Read the model definition and answer for the solid it produces. Units are mm, in the model's axes. Face numbers are marked on the shaded views. A direction names the side the tool comes from. Give positions to 0.01 mm unless a question says otherwise; leave off trailing zeros. Write each loop counter-clockwise with the first axis right and the second up, starting at its lowest first coordinate (ties: lowest second). Pieces come first, ordered by that corner, then holes. Notation, with made-up numbers: (85, -31) -> (131, -31) arc R5 ccw to (131, -22) -> close; hole circle Ø2 at (-27.5, 12.25). An arc over 180 degrees is marked (long way). Answer as CSV lines item,"result". Start each with the question number.
1. Given pin 1 (3 mm diameter, centred on x = 17.5, y = -2, fed in from +Z); pin 2 (1 mm diameter, centred on x = -26, z = -35.5, fed in from -Y); pin 3 (2 mm diameter, centred on y = -30.5, z = -18, fed in from +X); pin 4 (5 mm diameter, centred on x = 1, y = -1, fed in from -Z), each flat-ended and moving along its own axis, determine where each tip first touches the part or whether it passes through.
2. The part is cut by section A-A, the plane z = -35. Determine the outline of the cut face in (x, y).
3. A tool of negligible diameter and unlimited length cuts with its end or side. For the marked faces 1, 2 and 3, from which of +Z, -Z, +X, -X, +Y, -Y can it reach the whole face along a straight path? Write none if from no direction.
4. The part is cut by section B-B, the plane x = 0. Give the number of separate pieces and of enclosed holes in the cut face, and give its area (3 significant figures).
5. For a pull along Y with two mould halves and no side action, classify the marked faces 4, 5 and 6 as pulls with the +Y half, pulls with the -Y half, needs draft (parallel to the pull), parting line crosses it, or undercut.
6. Find the intervals of material crossed by line 1 (Y direction, x = 0, z = -42.05) (3 decimals); line 2 (Y direction, x = 0, z = -45.2); line 3 (X direction, y = 6.5, z = -10), in increasing order.
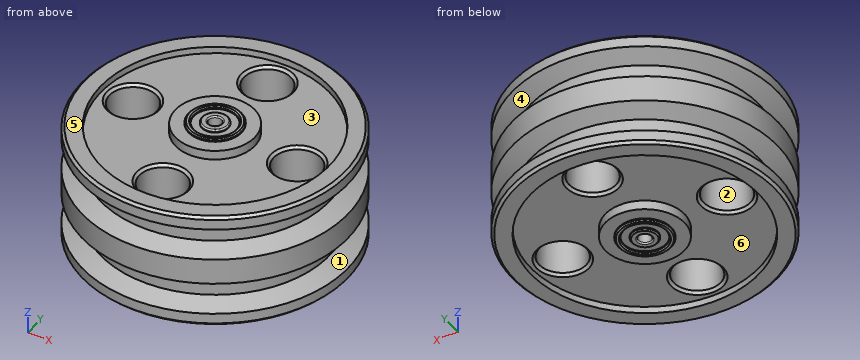
from build123d import *

# Parameters (mm, degrees)
SKETCH2_R            = 50.165
BOSS_EXTRUDE1_DEPTH  = 10
SKETCH4_R            = 43.18
BOSS_EXTRUDE2_DEPTH  = 2
SKETCH5_R            = 50.165
BOSS_EXTRUDE3_DEPTH  = 20
SKETCH7_R            = 43.18
BOSS_EXTRUDE4_DEPTH  = 2
SKETCH8_R            = 50.165
BOSS_EXTRUDE5_DEPTH  = 10
CHAMFER1_SIZE        = 14
CHAMFER1_SIZE_2      = 5.09558328
CHAMFER2_SIZE        = 5.09558328
CHAMFER2_SIZE_2      = 14
CHAMFER4_SIZE        = 14
CHAMFER4_SIZE_2      = 5.09558328
CHAMFER5_SIZE        = 5.09558328
CHAMFER5_SIZE_2      = 14
SKETCH13_R           = 43.18
CUT_EXTRUDE3_DEPTH   = 2.54
SKETCH18_R           = 15
BOSS_EXTRUDE12_DEPTH = 3.5
SKETCH19_R           = 10
BOSS_EXTRUDE13_DEPTH = 1
SKETCH20_R           = 8
SKETCH20_R_2         = 5
CUT_EXTRUDE4_DEPTH   = 1
CUT_EXTRUDE5_START   = -2.54
SKETCH22_R           = 43.18
SKETCH22_R_2         = 15
CUT_EXTRUDE5_DEPTH   = 2.54
SKETCH23_R           = 15
BOSS_EXTRUDE14_DEPTH = 1
BOSS_EXTRUDE15_START = 1
SKETCH24_R           = 10
BOSS_EXTRUDE15_DEPTH = 1
CUT_EXTRUDE6_START   = -1
SKETCH25_R           = 8
SKETCH25_R_2         = 5
CUT_EXTRUDE6_DEPTH   = 1
SKETCH26_R           = 2.5
CUT_EXTRUDE7_DEPTH   = 86.634199068
CHAMFER9_SIZE        = 0.5
FILLET1_R            = 0.5
FILLET2_R            = 0.5
CHAMFER10_SIZE       = 0.5
CHAMFER11_SIZE       = 0.5
FILLET3_R            = 0.5
SKETCH29_R           = 8.89
CUT_EXTRUDE9_DEPTH   = 85.530326215
CHAMFER12_SIZE       = 1
CHAMFER13_SIZE       = 1


with BuildPart() as part:
    # Sketch2 → Boss-Extrude1 (new body)
    with BuildSketch(Plane.XY):
        Circle(SKETCH2_R)
    extrude(amount=-BOSS_EXTRUDE1_DEPTH)

    # Sketch4 → Boss-Extrude2 (add)
    with BuildSketch(Plane(origin=(0, 0, -10), x_dir=(-1, 0, 0), z_dir=(0, 0, -1))):
        with Locations(Location((0, 0, 0), (0, 0, 180))):
            Circle(SKETCH4_R)
    extrude(amount=BOSS_EXTRUDE2_DEPTH)

    # Sketch5 → Boss-Extrude3 (add)
    with BuildSketch(Plane(origin=(0, 0, -12), x_dir=(-1, 0, 0), z_dir=(0, 0, -1))):
        with Locations(Location((0, 0, 0), (0, 0, 180))):
            Circle(SKETCH5_R)
    extrude(amount=BOSS_EXTRUDE3_DEPTH)

    # Sketch7 → Boss-Extrude4 (add)
    with BuildSketch(Plane(origin=(0, 0, -32), x_dir=(-1, 0, 0), z_dir=(0, 0, -1))):
        with Locations(Location((0, 0, 0), (0, 0, 180))):
            Circle(SKETCH7_R)
    extrude(amount=BOSS_EXTRUDE4_DEPTH)

    # Sketch8 → Boss-Extrude5 (add)
    with BuildSketch(Plane(origin=(0, 0, -34), x_dir=(-1, 0, 0), z_dir=(0, 0, -1))):
        with Locations(Location((0, 0, 0), (0, 0, 180))):
            Circle(SKETCH8_R)
    extrude(amount=BOSS_EXTRUDE5_DEPTH)

    # Chamfer1
    # the kernel refuses this chamfer: 14, 5.09558328 mm, written as the material it takes off along each edge
    with BuildSketch(Plane(origin=(0, 0, -10), x_dir=(1, 0, 0), z_dir=(0, -1, 0))) as chamfer1_piece_1_section:
        Polygon((50.165 - CHAMFER1_SIZE, 0), (50.165, CHAMFER1_SIZE_2), (50.165, 0), align=None)
    chamfer1_piece_1 = revolve(axis=Axis((0, 0, -10), (0, 0, 1)), mode=Mode.PRIVATE)
    chamfer1_piece_1 = chamfer1_piece_1 - Plane(origin=(0, 0, -6.275641512), x_dir=(1, 0, 0), z_dir=(0, 0, 1)) * Cylinder(43.18, 201, mode=Mode.PRIVATE)
    add(chamfer1_piece_1, mode=Mode.SUBTRACT)

    # Chamfer2
    # the kernel refuses this chamfer: 14, 5.09558328 mm, written as the material it takes off along each edge
    with BuildSketch(Plane(origin=(0, 0, -12), x_dir=(1, 0, 0), z_dir=(0, 1, 0))) as chamfer2_piece_1_section:
        Polygon((50.165, CHAMFER2_SIZE), (50.165 - CHAMFER2_SIZE_2, 0), (50.165, 0), align=None)
    chamfer2_piece_1 = revolve(axis=Axis((0, 0, -12), (0, 0, -1)), mode=Mode.PRIVATE)
    chamfer2_piece_1 = chamfer2_piece_1 - Plane(origin=(0, 0, -15.724358488), x_dir=(1, 0, 0), z_dir=(0, 0, 1)) * Cylinder(43.18, 201, mode=Mode.PRIVATE)
    add(chamfer2_piece_1, mode=Mode.SUBTRACT)

    # Chamfer4
    # the kernel refuses this chamfer: 14, 5.09558328 mm, written as the material it takes off along each edge
    with BuildSketch(Plane(origin=(0, 0, -32), x_dir=(1, 0, 0), z_dir=(0, 1, 0))) as chamfer4_piece_1_section:
        Polygon((50.165 - CHAMFER4_SIZE, 0), (50.165, -CHAMFER4_SIZE_2), (50.165, 0), align=None)
    chamfer4_piece_1 = revolve(axis=Axis((0, 0, -32), (0, 0, -1)), mode=Mode.PRIVATE)
    chamfer4_piece_1 = chamfer4_piece_1 - Plane(origin=(0, 0, -28.275641512), x_dir=(1, 0, 0), z_dir=(0, 0, 1)) * Cylinder(43.18, 201, mode=Mode.PRIVATE)
    add(chamfer4_piece_1, mode=Mode.SUBTRACT)

    # Chamfer5
    # the kernel refuses this chamfer: 14, 5.09558328 mm, written as the material it takes off along each edge
    with BuildSketch(Plane(origin=(0, 0, -34), x_dir=(1, 0, 0), z_dir=(0, 1, 0))) as chamfer5_piece_1_section:
        Polygon((50.165, CHAMFER5_SIZE), (50.165 - CHAMFER5_SIZE_2, 0), (50.165, 0), align=None)
    chamfer5_piece_1 = revolve(axis=Axis((0, 0, -34), (0, 0, -1)), mode=Mode.PRIVATE)
    chamfer5_piece_1 = chamfer5_piece_1 - Plane(origin=(0, 0, -37.724358488), x_dir=(1, 0, 0), z_dir=(0, 0, 1)) * Cylinder(43.18, 201, mode=Mode.PRIVATE)
    add(chamfer5_piece_1, mode=Mode.SUBTRACT)

    # Sketch13 → Cut-Extrude3 (cut)
    with BuildSketch(Plane.XY):
        Circle(SKETCH13_R)
    extrude(amount=-CUT_EXTRUDE3_DEPTH, mode=Mode.SUBTRACT)

    # Sketch18 → Boss-Extrude12 (add)
    with BuildSketch(Plane.XY.offset(-2.54)):
        Circle(SKETCH18_R)
    extrude(amount=BOSS_EXTRUDE12_DEPTH)

    # Sketch19 → Boss-Extrude13 (add)
    with BuildSketch(Plane.XY.offset(0.96)):
        Circle(SKETCH19_R)
    extrude(amount=BOSS_EXTRUDE13_DEPTH)

    # Sketch20 → Cut-Extrude4 (cut)
    with BuildSketch(Plane.XY.offset(1.96)):
        Circle(SKETCH20_R)
        Circle(SKETCH20_R_2, mode=Mode.SUBTRACT)
    extrude(amount=-CUT_EXTRUDE4_DEPTH, mode=Mode.SUBTRACT)

    # Sketch22 → Cut-Extrude5 (cut)
    with BuildSketch(Plane(origin=(0, 0, -44), x_dir=(-1, 0, 0), z_dir=(0, 0, -1)).offset(CUT_EXTRUDE5_START)):
        with Locations(Location((0, 0, 0), (0, 0, 180))):
            Circle(SKETCH22_R)
        with Locations(Location((0, 0, 0), (0, 0, 180))):
            Circle(SKETCH22_R_2, mode=Mode.SUBTRACT)
    extrude(amount=CUT_EXTRUDE5_DEPTH, mode=Mode.SUBTRACT)

    # Sketch23 → Boss-Extrude14 (add)
    with BuildSketch(Plane(origin=(0, 0, -44), x_dir=(-1, 0, 0), z_dir=(0, 0, -1))):
        with Locations(Location((0, 0, 0), (0, 0, 180))):
            Circle(SKETCH23_R)
    extrude(amount=BOSS_EXTRUDE14_DEPTH)

    # Sketch24 → Boss-Extrude15 (add)
    with BuildSketch(Plane(origin=(0, 0, -45), x_dir=(-1, 0, 0), z_dir=(0, 0, -1)).offset(BOSS_EXTRUDE15_START)):
        with Locations(Location((0, 0, 0), (0, 0, 180))):
            Circle(SKETCH24_R)
    extrude(amount=-BOSS_EXTRUDE15_DEPTH)

    # Sketch25 → Cut-Extrude6 (cut)
    with BuildSketch(Plane(origin=(0, 0, -46), x_dir=(-1, 0, 0), z_dir=(0, 0, -1)).offset(CUT_EXTRUDE6_START)):
        with Locations(Location((0, 0, 0), (0, 0, 180))):
            Circle(SKETCH25_R)
        with Locations(Location((0, 0, 0), (0, 0, 180))):
            Circle(SKETCH25_R_2, mode=Mode.SUBTRACT)
    extrude(amount=CUT_EXTRUDE6_DEPTH, mode=Mode.SUBTRACT)

    # Sketch26 → Cut-Extrude7 (cut, through all)
    with BuildSketch(Plane.XY.offset(1.96)):
        Circle(SKETCH26_R)
    extrude(amount=-CUT_EXTRUDE7_DEPTH, mode=Mode.SUBTRACT)

    # Chamfer9
    chamfer9_edges = [part.edges().sort_by_distance(p)[0] for p in [
        (-10, 0, 1.96),
        (-8, 0, 1.96),
    ]]
    chamfer(chamfer9_edges, length=CHAMFER9_SIZE)

    # Fillet1
    fillet1_edges = [part.edges().sort_by_distance(p)[0] for p in [
        (-5, 0, 1.96),
    ]]
    fillet(fillet1_edges, radius=FILLET1_R)

    # Fillet2
    fillet2_edges = [part.edges().sort_by_distance(p)[0] for p in [
        (-2.5, 0, 1.96),
    ]]
    fillet(fillet2_edges, radius=FILLET2_R)

    # Chamfer10
    chamfer10_edges = [part.edges().sort_by_distance(p)[0] for p in [
        (-10, 0, -46),
        (-8, 0, -46),
    ]]
    chamfer(chamfer10_edges, length=CHAMFER10_SIZE)

    # Chamfer11
    chamfer11_edges = [part.edges().sort_by_distance(p)[0] for p in [
        (-5, 0, -46),
    ]]
    chamfer(chamfer11_edges, length=CHAMFER11_SIZE)

    # Fillet3
    fillet3_edges = [part.edges().sort_by_distance(p)[0] for p in [
        (-2.5, 0, -46),
    ]]
    fillet(fillet3_edges, radius=FILLET3_R)

    # Sketch29 → Cut-Extrude9 (cut, through all)
    with BuildSketch(Plane(origin=(0, 0, -44), x_dir=(-1, 0, 0), z_dir=(0, 0, -1))):
        with Locations((0, 31.75)):
            Circle(SKETCH29_R)
        with Locations((31.75, 0)):
            Circle(SKETCH29_R)
        with Locations((0, -31.75)):
            Circle(SKETCH29_R)
        with Locations((-31.75, 0)):
            Circle(SKETCH29_R)
    extrude(amount=-CUT_EXTRUDE9_DEPTH, mode=Mode.SUBTRACT)

    # Chamfer12
    chamfer12_edges = [part.edges().sort_by_distance(p)[0] for p in [
        (8.89, 31.75, -2.54),
        (8.89, 31.75, -41.46),
        (-22.86, 0, -2.54),
        (-22.86, 0, -41.46),
        (8.89, -31.75, -2.54),
        (8.89, -31.75, -41.46),
        (40.64, 0, -2.54),
        (40.64, 0, -41.46),
    ]]
    chamfer(chamfer12_edges, length=CHAMFER12_SIZE)

    # Chamfer13
    chamfer13_edges = [part.edges().sort_by_distance(p)[0] for p in [
        (-50.165, 0, 0),
        (-50.165, 0, -44),
    ]]
    chamfer(chamfer13_edges, length=CHAMFER13_SIZE)


solid = part.part
Results found:
1,pin 1,"stops at z = -2.54"
1,pin 2,"stops at y = -34.85"
1,pin 3,"stops at x = 40.57"
1,pin 4,"stops at z = -46"
2,outline,"circle Ø86.36 at (0, 0); hole circle Ø17.78 at (-31.75, 0); hole circle Ø17.78 at (0, -31.75); hole circle Ø17.78 at (0, 31.75); hole circle Ø5 at (0, 0); hole circle Ø17.78 at (31.75, 0)"
3,face 1,"none"
3,face 2,"+Z, -Z"
3,face 3,"+Z"
4,separate pieces,"4"
4,enclosed holes,"0"
4,area,"2,310 mm²"
5,face 4,"parting line crosses it"
5,face 5,"needs draft"
5,face 6,"undercut"
6,line 1,"y = -50.165 to -43.18, -15 to -2.5, 2.5 to 15, 43.18 to 50.165"
6,line 2,"y = -10 to -8, -5 to -2.5, 2.5 to 5, 8 to 10"
6,line 3,"x = -42.69 to -37.81, -25.69 to 25.69, 37.81 to 42.69"
